from build123d import *

# Parameters (mm, degrees)
PAD_DEPTH    = 12
SKETCH001_R  = 2.1
POCKET_DEPTH = 9.501
FILLET_R     = 3
FILLET001_R  = 3


with BuildPart() as part:
    # Sketch → Pad (new body)
    with BuildSketch(Plane.XY):
        with BuildLine():
            ThreePointArc((-0.25, -3.741657), (2.738613, 2.561738), (-3.75, 0))
            Line((-3.75, -16), (-3.75, 0))
            Line((-6.75, -16), (-3.75, -16))
            Line((-6.75, 0), (-6.75, -16))
            ThreePointArc((2.75, -6.164414), (3.674235, 5.662376), (-6.75, 0))
            Line((2.75, -16), (2.75, -6.164414))
            Line((-0.25, -16), (2.75, -16))
            Line((-0.25, -3.741657), (-0.25, -16))
        make_face()
    extrude(amount=PAD_DEPTH)

    # Sketch001 → Pocket (cut, through all)
    with BuildSketch(Plane.YZ.offset(2.75)):
        with Locations((-11, 6)):
            Circle(SKETCH001_R)
    extrude(amount=-POCKET_DEPTH, mode=Mode.SUBTRACT)

    # Fillet
    fillet_edges = [part.edges().sort_by_distance(p)[0] for p in [
        (1.25, -16, 0),
        (-5.25, -16, 0),
    ]]
    fillet(fillet_edges, radius=FILLET_R)

    # Fillet001
    fillet001_edges = [part.edges().sort_by_distance(p)[0] for p in [
        (-5.25, -16, 12),
        (1.25, -16, 12),
    ]]
    fillet(fillet001_edges, radius=FILLET001_R)


solid = part.part
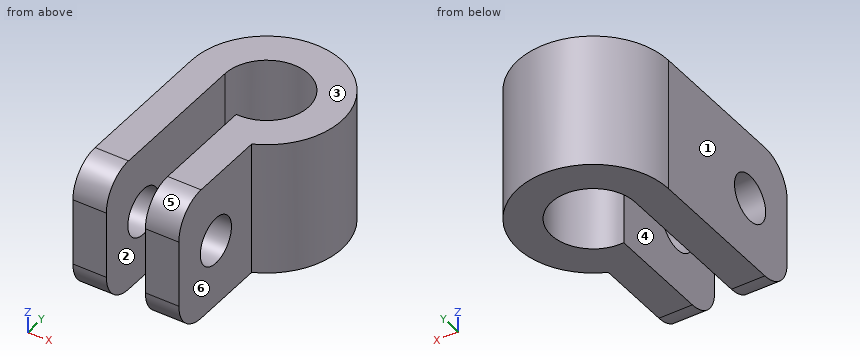
Build history of the part. All positions in model axes, mm. Face numbers are marked on the shaded views. A direction names the side the tool comes from. Give positions to 0.01 mm unless a question says otherwise; leave off trailing zeros. Order: outer loops, then holes, each group sorted by start corner. A loop starts at its lowest first (then second) coordinate and runs counter-clockwise, first axis right, second up. Notation, with made-up numbers: M 38,-19.75 L 87,-19.75 A18 ccw 87,-8.75 Z; hole C 36,45.5 d1. An arc over 180 degrees is marked long. Put each result on its own line as item: value.
Item 1: Wall check: probe 1 along X at (y, z) = (-12.75, 8.5); probe 2 along Z at (x, y) = (-4.35, -11); probe 3 along Y at (x, z) = (1.5, 2.25). Give the ranges that are in metal, low to high.
Results are:
probe 1: -6.75 to -3.75, -0.25 to 2.75
probe 2: 0 to 3.9, 8.1 to 12
probe 3: -15.9 to -3.44, 3.44 to 6.58
Item 2: Cut at C-C on y = -0.75. Write the cut outline in (x, z).
Results are:
outline: M -6.75,0 L -3.75,0 L -3.75,12 L -6.75,12 Z; M 3.67,0 L 6.71,0 L 6.71,12 L 3.67,12 Z
Item 3: Drop flat-ended pins along their axis: pin 1 Ø6 at (y, z) = (-13, 4) entering from +X; pin 2 Ø2 at (y, z) = (2, 5.5) entering from -X; pin 3 Ø1.5 at (y, z) = (3.5, 5) entering from +X; pin 4 Ø3.5 at (y, z) = (-11, 6) entering from +X. Give the stop position or say it passes through.
Results are:
pin 1: x = 2.75
pin 2: x = -6.68
pin 3: x = 6.16
pin 4: through
Item 4: Cut at D-D on y = -12. Write the cut outline in (x, z), then the cut area to 3 significant figures.
Results are:
outline: M -6.75,0 L -3.75,0 L -3.75,4.15 L -6.75,4.15 Z; M -6.75,7.85 L -3.75,7.85 L -3.75,12 L -6.75,12 Z; M -0.25,0 L 2.75,0 L 2.75,4.15 L -0.25,4.15 Z; M -0.25,7.85 L 2.75,7.85 L 2.75,12 L -0.25,12 Z
area: 49.8 mm2
Item 5: Cut at B-B on z = 6. Write the cut outline in (x, y).
Results are:
outline: M -6.75,-16 L -3.75,-16 L -3.75,-13.1 L -6.75,-13.1 Z; M -6.75,-8.9 L -3.75,-8.9 L -3.75,0 A3.75 cw long -0.25,-3.74 L -0.25,-8.9 L 2.75,-8.9 L 2.75,-6.16 A6.75 ccw long -6.75,0 Z; M -0.25,-16 L 2.75,-16 L 2.75,-13.1 L -0.25,-13.1 Z
Item 6: Which spindle directions (+Z, -Z, +X, -X, +Y, -Y) get a long thin tool onto all of the face, cutting with end or side? Do the marked faces 4, 5 and 6. Say none if no direction does.
Results are:
face 4: +Z, -Z, -Y
face 5: +Z, +X, -X, -Y
face 6: +Z, -Z, +X, -Y
Item 7: Pull direction X, two halves, no side cores. Call the marked faces 1, 2 and 3: +X half, -X half, draft (parallel to the pull), parting line (faces both ways), or undercut.
Results are:
face 1: -X half
face 2: undercut
face 3: draft
Item 8: Cut at A-A on x = 0. Write the cut outline in (y, z).
Results are:
outline: M -16,3 A3 ccw -13,0 L -3.75,0 L -3.75,12 L -13,12 A3 ccw -16,9 Z; M 3.75,0 L 6.75,0 L 6.75,12 L 3.75,12 Z; hole C -11,6 d4.2
